from build123d import *

# Parameters (mm, degrees)
BOX061_W               = 37
BOX061_H               = 160
BOX061_DEPTH           = 120
BOX061_PITCH_ANGLE     = -15
BOX060_W               = 37.35
BOX060_H               = 160
BOX060_DEPTH           = 120
BOX060_PITCH_ANGLE     = -15
BOX062_W               = 64
BOX062_H               = 5
BOX062_DEPTH           = 37
CYLINDER059_R          = 0.8
CYLINDER059_DEPTH      = 9
CYLINDER059_ROLL_ANGLE = 90
CYLINDER060_R          = 0.8
CYLINDER060_DEPTH      = 9
CYLINDER060_ROLL_ANGLE = 90
CYLINDER061_R          = 0.8
CYLINDER061_DEPTH      = 9
CYLINDER061_ROLL_ANGLE = 90
CYLINDER062_R          = 0.8
CYLINDER062_DEPTH      = 9
CYLINDER062_ROLL_ANGLE = 90
BOX067_W               = 37
BOX067_H               = 160
BOX067_DEPTH           = 120
BOX067_PITCH_ANGLE     = -15
BOX066_W               = 37.35
BOX066_H               = 160
BOX066_DEPTH           = 120
BOX066_PITCH_ANGLE     = -15
BOX065_W               = 76
BOX065_H               = 3
BOX065_DEPTH           = 50
FILLET007_R            = 2
CHAMFER004_SIZE        = 3


with BuildPart() as cube033:
    # Box061 → Box061 (new body)
    with BuildSketch(Plane.XY):
        with Locations((18.5, 80)):
            Rectangle(BOX061_W, BOX061_H)
    extrude(amount=BOX061_DEPTH)


with BuildPart() as cube033_1:
    # Box061 pitch: moved
    add(cube033.part.rotate(Axis((0, 0, 0), (0, 1, 0)), BOX061_PITCH_ANGLE))


with BuildPart() as cube033_2:
    # Box061 placement: moved
    add(cube033_1.part.moved(Location((549, -50, -4))))


with BuildPart() as fusion056:
    # Box060 → Box060 (new body)
    with BuildSketch(Plane.XY):
        with Locations((18.675, 80)):
            Rectangle(BOX060_W, BOX060_H)
    extrude(amount=BOX060_DEPTH)


with BuildPart() as fusion056_1:
    # Box060 pitch: moved
    add(fusion056.part.rotate(Axis((0, 0, 0), (0, 1, 0)), BOX060_PITCH_ANGLE))


with BuildPart() as fusion056_2:
    # Box060 placement: moved
    add(fusion056_1.part.moved(Location((470.94, -50, -10))))

    # Fusion056: union Cube033
    add(cube033_2.part)


with BuildPart() as cut078:
    # Box062 → Box062 (new body)
    with BuildSketch(Plane(origin=(468, -49, 68), x_dir=(1, 0, 0), z_dir=(0, 0, 1))):
        with Locations((32, 2.5)):
            Rectangle(BOX062_W, BOX062_H)
    extrude(amount=BOX062_DEPTH)

    # Cut078: cut Fusion056
    add(fusion056_2.part, mode=Mode.SUBTRACT)


with BuildPart() as cylinder059:
    # Cylinder059 → Cylinder059 (new body)
    with BuildSketch(Plane.XY):
        Circle(CYLINDER059_R)
    extrude(amount=CYLINDER059_DEPTH)


with BuildPart() as cylinder059_1:
    # Cylinder059 roll: moved
    add(cylinder059.part.rotate(Axis((0, 0, 0), (1, 0, 0)), CYLINDER059_ROLL_ANGLE))


with BuildPart() as cylinder059_2:
    # Cylinder059 placement: moved
    add(cylinder059_1.part.moved(Location((519.3, -40, 106))))


with BuildPart() as fusion061:
    # Cylinder060 → Cylinder060 (new body)
    with BuildSketch(Plane.XY):
        Circle(CYLINDER060_R)
    extrude(amount=CYLINDER060_DEPTH)


with BuildPart() as fusion061_1:
    # Cylinder060 roll: moved
    add(fusion061.part.rotate(Axis((0, 0, 0), (1, 0, 0)), CYLINDER060_ROLL_ANGLE))


with BuildPart() as fusion061_2:
    # Cylinder060 placement: moved
    add(fusion061_1.part.moved(Location((531, -40, 61))))

    # Fusion061: union Cylinder059
    add(cylinder059_2.part)


with BuildPart() as cylinder061:
    # Cylinder061 → Cylinder061 (new body)
    with BuildSketch(Plane.XY):
        Circle(CYLINDER061_R)
    extrude(amount=CYLINDER061_DEPTH)


with BuildPart() as cylinder061_1:
    # Cylinder061 roll: moved
    add(cylinder061.part.rotate(Axis((0, 0, 0), (1, 0, 0)), CYLINDER061_ROLL_ANGLE))


with BuildPart() as cylinder061_2:
    # Cylinder061 placement: moved
    add(cylinder061_1.part.moved(Location((519.3, -40, 106))))


with BuildPart() as fusion062:
    # Cylinder062 → Cylinder062 (new body)
    with BuildSketch(Plane.XY):
        Circle(CYLINDER062_R)
    extrude(amount=CYLINDER062_DEPTH)


with BuildPart() as fusion062_1:
    # Cylinder062 roll: moved
    add(fusion062.part.rotate(Axis((0, 0, 0), (1, 0, 0)), CYLINDER062_ROLL_ANGLE))


with BuildPart() as fusion062_2:
    # Cylinder062 placement: moved
    add(fusion062_1.part.moved(Location((531, -40, 61))))

    # Fusion063: union Cylinder061
    add(cylinder061_2.part)


with BuildPart() as fusion062_3:
    # Fusion063 placement: moved
    add(fusion062_2.part.moved(Location((-54, 0, 0))))

    # Fusion062: union Fusion061
    add(fusion061_2.part)


with BuildPart() as fusion062_4:
    # Fusion062 placement: moved
    add(fusion062_3.part.moved(Location((0, -1, 0))))


with BuildPart() as cube039:
    # Box067 → Box067 (new body)
    with BuildSketch(Plane.XY):
        with Locations((18.5, 80)):
            Rectangle(BOX067_W, BOX067_H)
    extrude(amount=BOX067_DEPTH)


with BuildPart() as cube039_1:
    # Box067 pitch: moved
    add(cube039.part.rotate(Axis((0, 0, 0), (0, 1, 0)), BOX067_PITCH_ANGLE))


with BuildPart() as cube039_2:
    # Box067 placement: moved
    add(cube039_1.part.moved(Location((551, -50, -4))))


with BuildPart() as fusion060:
    # Box066 → Box066 (new body)
    with BuildSketch(Plane.XY):
        with Locations((18.675, 80)):
            Rectangle(BOX066_W, BOX066_H)
    extrude(amount=BOX066_DEPTH)


with BuildPart() as fusion060_1:
    # Box066 pitch: moved
    add(fusion060.part.rotate(Axis((0, 0, 0), (0, 1, 0)), BOX066_PITCH_ANGLE))


with BuildPart() as fusion060_2:
    # Box066 placement: moved
    add(fusion060_1.part.moved(Location((453.94, -50, -10))))

    # Fusion060: union Cube039
    add(cube039_2.part)


with BuildPart() as left_back_door_mech_cover:
    # Box065 → Box065 (new body)
    with BuildSketch(Plane(origin=(460, -49, 58), x_dir=(1, 0, 0), z_dir=(0, 0, 1))):
        with Locations((38, 1.5)):
            Rectangle(BOX065_W, BOX065_H)
    extrude(amount=BOX065_DEPTH)

    # Cut063: cut Fusion060
    add(fusion060_2.part, mode=Mode.SUBTRACT)


with BuildPart() as left_back_door_mech_cover_1:
    # Cut063 placement: moved
    add(left_back_door_mech_cover.part.moved(Location((0, -1, 0))))

    # Cut064: cut Fusion062
    add(fusion062_4.part, mode=Mode.SUBTRACT)

    # Fillet007
    fillet007_edges = [left_back_door_mech_cover_1.edges().sort_by_distance(p)[0] for p in [
        (534.38715, -48.5, 58),
        (474.38702, -48.5, 58),
        (520.98969, -48.5, 108),
    ]]
    fillet(fillet007_edges, radius=FILLET007_R)

    # Chamfer004
    chamfer004_edges = [left_back_door_mech_cover_1.edges().sort_by_distance(p)[0] for p in [
        (460.989561, -48.5, 108),
    ]]
    chamfer(chamfer004_edges, length=CHAMFER004_SIZE)

    # Cut079: cut Cut078
    add(cut078.part, mode=Mode.SUBTRACT)


solid = left_back_door_mech_cover_1.part
Geometry check sheet. Reference: the model listing, model coordinates, mm. A direction names the side the tool comes from. Round coordinates to 2 decimals unless told otherwise and drop trailing zeros. Order: outer loops, then holes, each group sorted by start corner. A loop starts at its lowest first (then second) coordinate and runs counter-clockwise, first axis right, second up. Notation, with made-up numbers: M 56,-22 L 82,-22 A11 cw 82,-10 Z; hole C -35.75,-27 d9. An arc over 180 degrees is marked long. Write each question's results on one line, items separated by ' | '. Start each with the question number.
1. Cross-section at B-B on y = -48.15. Record the boundary of the cut face in (x, z).
2. Draft check along Z on faces 1 (the face through (467.963, -48.521, 81.973)), 2 (the face through (491, -48, 108)), 3 (the face through (483.82, -48.01, 86.24)), 4 (the face through (504, -49, 86)). Enter one of: pulls with the +Z half, pulls with the -Z half, needs draft (parallel to the pull), parting line crosses it, or undercut.
3. Go/stop test with flat-tipped pins: P1, Ø1, axis at x = 465.3, z = 106, coming from the -Y side; P2, Ø18.5, axis at x = 491.5, z = 94.5, coming from the +Y side. Record where each tip stops, or that it passes through.
4. Cross-section at A-A on x = 477. Record the boundary of the cut face in (y, z), plus the area to 3 significant figures.
5. Cross-section at C-C on x = 492. Record the boundary of the cut face in (y, z).
6. Set-up check for faces 5 (the face through (474.72, -48.52, 58.4)), 6 (the face through (524.82, -48.01, 86.24)): record each of +Z, -Z, +X, -X, +Y, -Y from which the full face is reachable in a straight line by a thin tool's end or side.
7. Material ranges on L1, parallel to Z at x = 496, y = -48.3; L2, parallel to X at y = -48.65, z = 61; L3, parallel to X at y = -48.75, z = 106, recorded low to high. Write a range as from..to.
8. Cross-section at D-D on z = 83.5. Record the boundary of the cut face in (x, y), plus the area to 3 significant figures.
Resolved:
1) outline: M 461.77,105.1 L 473.99,59.48 A2 ccw 475.92,58 L 531.78,58 A2 ccw 533.71,60.52 L 521.39,106.52 A2 ccw 519.46,108 L 463.99,108 Z; hole C 465.3,106 d1.6; hole C 477,61 d1.6; hole M 478.79,105 L 488.71,68 L 529.71,68 L 519.79,105 Z; hole C 519.3,106 d1.6; hole C 531,61 d1.6
2) face 1: pulls with the -Z half | face 2: pulls with the +Z half | face 3: undercut | face 4: undercut
3) P1: through | P2: y = -49
4) outline: M -50,58 L -47,58 L -47,60.2 L -50,60.2 Z; M -50,61.8 L -47,61.8 L -47,108 L -50,108 Z | area: 145 mm2
5) outline: M -50,58 L -47,58 L -47,68 L -49,68 L -49,105 L -47,105 L -47,108 L -50,108 Z
6) face 5: -Z, -X, +Y, -Y | face 6: +Y
7) L1: 58..68, 105..108 | L2: 473.58..476.2, 477.8..530.2, 531.8..533.58 | L3: 462.45..464.5, 466.1..518.5, 520.1..521.53
8) outline: M 467.55,-50 L 527.55,-50 L 527.55,-47 L 525.55,-47 L 525.55,-49 L 484.55,-49 L 484.55,-47 L 467.55,-47 Z | area: 98.0 mm2
